Autodesk Inventor part; units mm, degrees
ref_plane "YZ Plane" through (0, 0, 0) normal (1, 0, 0) x (0, 1, 0)
ref_plane "XZ Plane" through (0, 0, 0) normal (0, 1, 0) x (-1, 0, 0)
ref_plane "XY Plane" through (0, 0, 0) normal (0, 0, 1) x (1, 0, 0)
sketch "Sketch1" plane through (0, 0, 0) normal (1, 0, 0) x (0, 1, 0)
  circle A0 centre (16, 0) radius 2
  circle A1 centre (-16, 0) radius 2
  line L0 (-21, 3) -> (21, 3)
  line L1 (21, 3) -> (21, -3)
  line L2 (21, -3) -> (-21, -3)
  line L3 (-21, -3) -> (-21, 3)
  line L4 (-21, 3) -> (21, -3) construction
  line L5 (21, 3) -> (-21, -3) construction
  point P0 (0, 0)
  dimension "d0" = 16
  dimension "d1" = 16
  dimension "d2" = 42
  dimension "d3" = 4
  dimension "d4" = 4
  dimension "d5" = 6
extrude "Extrusion1" add sketch "Sketch1" along normal blind 4.6
properties part number "BearingBlockSpacer"
Design review of the part built by this model. Coordinates are the model's own, in mm. Coordinates: 2 decimals unless noted, no trailing zeros. Write each loop counter-clockwise with the first axis right and the second up, starting at its lowest first coordinate (ties: lowest second). Pieces come first, ordered by that corner, then holes.
1) Add section C-C (x = 3.55). Write out the cut boundary in (y, z), plus the area to 3 significant figures.
2) Mouldability with a two-part tool opening along Z and no side actions: class faces 1 (the flat face through (2, 0, -3)), 2 (the cylindrical face through (2.3, 14.4, 1.2)), 3 (the flat face through (2, -21, 0)) as +Z half, -Z half, draft (parallel to the pull), parting line (faces both ways), or undercut.
3) Add section A-A (z = 0). Write out the cut boundary in (x, y), plus the area to 3 significant figures.
4) Add section B-B (y = -16). Write out the cut boundary in (x, z), plus the area to 3 significant figures.
5) To check wall thickness, follow L1, parallel to Z at x = 3.4, y = -16; L2, parallel to Y at x = 1.7, z = -1.8; L3, parallel to Y at x = 3.8, z = 1.4. State the ranges of each line that lie inside material, in increasing order.
Check result:
1. outline: (-21, -3) - (21, -3) - (21, 3) - (-21, 3) - close; hole circle Ø4 at (-16, 0); hole circle Ø4 at (16, 0)
1. area: 227 mm2
2. face 1: -Z half
2. face 2: undercut
2. face 3: draft
3. outline: (0, -21) - (4.6, -21) - (4.6, -18) - (0, -18) - close; (0, -14) - (4.6, -14) - (4.6, 14) - (0, 14) - close; (0, 18) - (4.6, 18) - (4.6, 21) - (0, 21) - close
3. area: 156 mm2
4. outline: (0, -3) - (4.6, -3) - (4.6, -2) - (0, -2) - close; (0, 2) - (4.6, 2) - (4.6, 3) - (0, 3) - close
4. area: 9.20 mm2
5. L1: z = -3 to -2, 2 to 3
5. L2: y = -21 to -16.87, -15.13 to 15.13, 16.87 to 21
5. L3: y = -21 to -17.43, -14.57 to 14.57, 17.43 to 21
